Work out the finished part from the listing and answer in its coordinate system (mm). Face numbers are marked on the shaded views. Round coordinates to 2 decimals unless told otherwise and drop trailing zeros. Order: outer loops, then holes, each group sorted by start corner. A loop starts at its lowest first (then second) coordinate and runs counter-clockwise, first axis right, second up. Notation, with made-up numbers: (36, 44) - (53, 44) arc R25 cw to (53, 76) - close; hole circle Ø2 at (37.5, -11.75). An arc over 180 degrees is marked (long way). Use one line per item in the form item = value. Start each with the question number.
Q1. For a pull along X with two mould halves and no side action, classify the marked faces 1, 2 and 3 as +X half, -X half, draft (parallel to the pull), parting line (faces both ways), or undercut.
Q2. The part is cut by section B-B on z = 4.75. Determine the outline of the cut face in (x, y).
Q3. The part is cut by section A-A on y = -25.4. Determine the outline of the cut face in (x, z), plus the area to 3 significant figures.
Q4. Find the intervals of material crossed by line 1 (Y direction, x = -25.4, z = 11.2); line 2 (Y direction, x = 0, z = 5.25); line 3 (X direction, y = 25, z = 10.5), in increasing order. Write a range as [from, to].
Q5. Given P1, Ø4.5, axis at x = -25.4, y = 25.4, coming from the +Z side, flat-ended and moving along its own axis, determine where the tip first touches the part or whether it passes through.
Q6. The part is cut by section C-C on x = 0. Determine the outline of the cut face in (y, z).
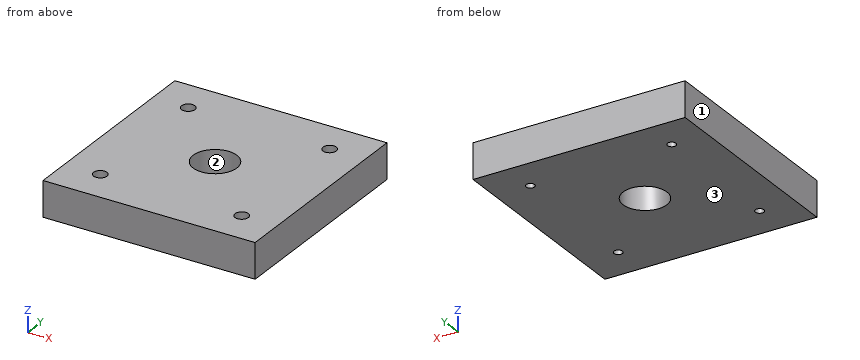
from build123d import *

# Parameters (mm, degrees)
SKETCH2_W           = 76.2
SKETCH2_H           = 76.2
SKETCH2_R           = 7.874
BOSS_EXTRUDE1_DEPTH = 12.7
SKETCH6_R           = 2.413
CUT_EXTRUDE3_DEPTH  = 3.048
SKETCH7_R           = 1.524
CUT_EXTRUDE4_DEPTH  = 55.739209932


with BuildPart() as part:
    # Sketch2 → Boss-Extrude1 (new body)
    with BuildSketch(Plane.XY):
        Rectangle(SKETCH2_W, SKETCH2_H)
        Circle(SKETCH2_R, mode=Mode.SUBTRACT)
    extrude(amount=BOSS_EXTRUDE1_DEPTH)

    # Sketch6 → Cut-Extrude3 (cut)
    with BuildSketch(Plane.XY.offset(12.7)):
        with Locations((-25.4, 25.4)):
            Circle(SKETCH6_R)
        with Locations((25.4, 25.4)):
            Circle(SKETCH6_R)
        with Locations((25.4, -25.4)):
            Circle(SKETCH6_R)
        with Locations((-25.4, -25.4)):
            Circle(SKETCH6_R)
    extrude(amount=-CUT_EXTRUDE3_DEPTH, mode=Mode.SUBTRACT)

    # Sketch7 → Cut-Extrude4 (cut, through all)
    with BuildSketch(Plane.XY.offset(9.652)):
        with Locations((-25.4, 25.4)):
            Circle(SKETCH7_R)
        with Locations((25.4, 25.4)):
            Circle(SKETCH7_R)
        with Locations((25.4, -25.4)):
            Circle(SKETCH7_R)
        with Locations((-25.4, -25.4)):
            Circle(SKETCH7_R)
    extrude(amount=-CUT_EXTRUDE4_DEPTH, mode=Mode.SUBTRACT)


solid = part.part
Found:
q1.face_1 = -X half
q1.face_2 = undercut
q1.face_3 = draft
q2.outline = (-38.1, -38.1) - (38.1, -38.1) - (38.1, 38.1) - (-38.1, 38.1) - close; hole circle Ø3.05 at (-25.4, -25.4); hole circle Ø3.05 at (-25.4, 25.4); hole circle Ø15.75 at (0, 0); hole circle Ø3.05 at (25.4, -25.4); hole circle Ø3.05 at (25.4, 25.4)
q3.outline = (-38.1, 0) - (-26.92, 0) - (-26.92, 9.65) - (-27.81, 9.65) - (-27.81, 12.7) - (-38.1, 12.7) - close; (-23.88, 0) - (23.88, 0) - (23.88, 9.65) - (22.99, 9.65) - (22.99, 12.7) - (-22.99, 12.7) - (-22.99, 9.65) - (-23.88, 9.65) - close; (26.92, 0) - (38.1, 0) - (38.1, 12.7) - (27.81, 12.7) - (27.81, 9.65) - (26.92, 9.65) - close
q3.area = 879 mm²
q4.line_1 = [-38.1, -27.81], [-22.99, 22.99], [27.81, 38.1]
q4.line_2 = [-38.1, -7.87], [7.87, 38.1]
q4.line_3 = [-38.1, -27.78], [-23.02, 23.02], [27.78, 38.1]
q5.P1 = 9.65
q6.outline = (-38.1, 0) - (-7.87, 0) - (-7.87, 12.7) - (-38.1, 12.7) - close; (7.87, 0) - (38.1, 0) - (38.1, 12.7) - (7.87, 12.7) - close
